from build123d import *

# Parameters (mm, degrees)
F2_W     = 20
F2_H     = 20
F3_DEPTH = 450
F4_R     = 3
F5_T     = -2


with BuildPart() as f3:
    # F2 (on Front) → F3 (new body, symmetric)
    with BuildSketch(Plane.XZ):
        Rectangle(F2_W, F2_H)
    extrude(amount=F3_DEPTH, both=True)

    # F4
    f4_edges = [f3.edges().sort_by_distance(p)[0] for p in [
        (10, 0, 10),
        (-10, 0, 10),
        (10, 0, -10),
        (-10, 0, -10),
    ]]
    fillet(f4_edges, radius=F4_R)

    # F5
    f5_openings = [f3.faces().sort_by_distance(p)[0] for p in [
        (0, -450, 0),
        (0, 450, 0),
    ]]
    offset(amount=F5_T, openings=f5_openings)


solid = f3.part
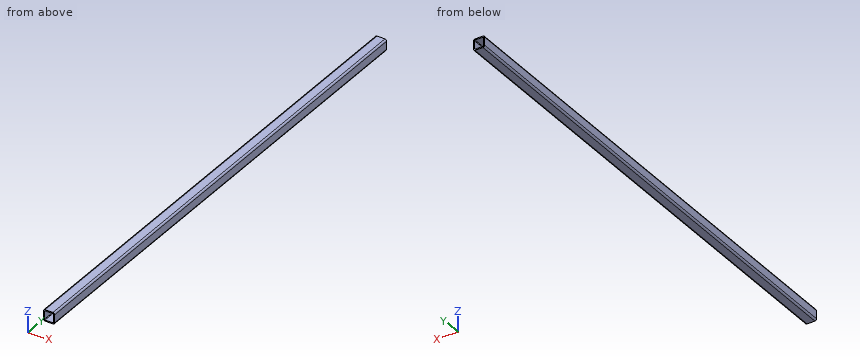
Read the model definition and answer for the solid it produces. Units are mm, in the model's axes. Coordinates: 2 decimals unless noted, no trailing zeros. Loops run counter-clockwise (first coordinate to the right, second up) from the corner with the lowest first, then second, coordinate; pieces in that order, holes last. Notation, with made-up numbers: (-14.5, -19.75) - (34.5, -19.75) arc R22 ccw to (34.5, 10.25) - close; hole circle Ø6 at (89.25, -11). An arc over 180 degrees is marked (long way). Answer in a Markdown table with one row per item.
Q1. Find section A-A on x = 1.25. Write down the section's boundary in (y, z).
Here are the results:
| item | result |
|---|---|
| outline | (-450, -10) - (450, -10) - (450, -8) - (-450, -8) - close; (-450, 8) - (450, 8) - (450, 10) - (-450, 10) - close |
Q2. Find section C-C on y = -172. Write down the section's boundary in (x, z), plus the area to 3 significant figures.
Here are the results:
| item | result |
|---|---|
| outline | (-10, -7) arc R3 ccw to (-7, -10) - (7, -10) arc R3 ccw to (10, -7) - (10, 7) arc R3 ccw to (7, 10) - (-7, 10) arc R3 ccw to (-10, 7) - close; hole (-8, -7) arc R1 ccw to (-7, -8) - (7, -8) arc R1 ccw to (8, -7) - (8, 7) arc R1 ccw to (7, 8) - (-7, 8) arc R1 ccw to (-8, 7) - close |
| area | 137 mm^2 |
Q3. Find section B-B on z = -2.25. Write down the section's boundary in (x, y).
Here are the results:
| item | result |
|---|---|
| outline | (-10, -450) - (-8, -450) - (-8, 450) - (-10, 450) - close; (8, -450) - (10, -450) - (10, 450) - (8, 450) - close |
Q4. Straight lines are drawn through the part: line 1 along X through (y, z) = (-103.5, 2); line 2 along X through (y, z) = (-78.5, -7.5). For each, find the intervals that lie inside material, in ascending order. Write a range as [from, to].
Here are the results:
| item | result |
|---|---|
| line 1 | x = [-10, -8], [8, 10] |
| line 2 | x = [-9.96, -7.87], [7.87, 9.96] |
